Can you work these out from the drawing? Everything is in mm from the part's minimum corner. Round coordinates to 2 decimals unless told otherwise and drop trailing zeros. Write each loop counter-clockwise with the first axis right and the second up, starting at its lowest first coordinate (ties: lowest second). Pieces come first, ordered by that corner, then holes. Notation, with made-up numbers: M -28.5,13.25 L -24.5,13.25 A25 cw -24.5,43.25 Z; hole C 79,79.5 d1. An arc over 180 degrees is marked long. Use a Markdown table: item, result. Add a question column.
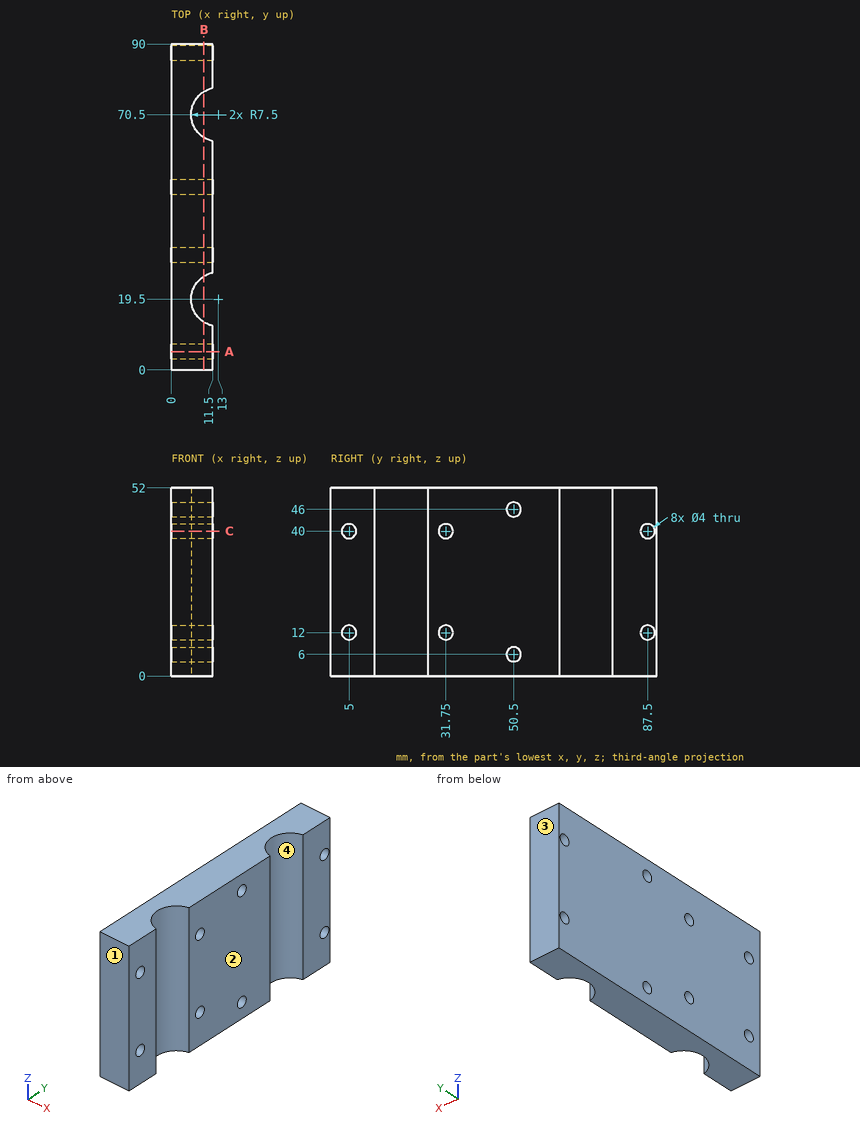
Item 1: Imagine slicing it at B-B on x = 9. Count the separate pieces of the cut face and the enclosed holes in it, plus the area to 3 significant figures.
Item 2: I need wall thicknesses on probe 1 along Z at (x, y) = (3.75, 50.5); probe 2 along Y at (x, z) = (11, 34); probe 3 along Y at (x, z) = (10.5, 34). Which ranges of each line are inside material? Lowest first, please. Write a range as from..to.
Item 3: Imagine slicing it at A-A on y = 5. List the corners of the cut face in (x, z) for me, plus the area to 3 significant figures.
Item 4: For pin 1 Ø1 at (y, z) = (69, 27) entering from +X, with a flat end and sliding along its axis, tell me the tip position at first contact or that it passes through.
Item 5: Imagine slicing it at C-C on z = 40. List the corners of the cut face in (x, y) for me.
Item 6: If we mould it in two halves opening along Y, with no side actions, what happens to the marked faces 1, 2, 3 and 4? For each: +Y half, -Y half, draft (parallel to the pull), parting line (faces both ways), or undercut.
The answers:
| question | item | result |
|---|---|---|
| 1 | separate pieces | 3 |
| 1 | enclosed holes | 8 |
| 1 | area | 3,260 mm² |
| 2 | probe 1 | 0..4, 8..44, 48..52 |
| 2 | probe 2 | 0..12.27, 26.73..63.27, 77.73..90 |
| 2 | probe 3 | 0..12.43, 26.57..63.43, 77.57..90 |
| 3 | outline | M 0,0 L 11.5,0 L 11.5,10 L 0,10 Z; M 0,14 L 11.5,14 L 11.5,38 L 0,38 Z; M 0,42 L 11.5,42 L 11.5,52 L 0,52 Z |
| 3 | area | 506 mm² |
| 4 | pin 1 | x = 5.77 |
| 5 | outline | M 0,0 L 11.5,0 L 11.5,3 L 0,3 Z; M 0,7 L 11.5,7 L 11.5,12.15 A7.5 cw 11.5,26.85 L 11.5,29.75 L 0,29.75 Z; M 0,33.75 L 11.5,33.75 L 11.5,63.15 A7.5 cw 11.5,77.85 L 11.5,85.5 L 0,85.5 Z; M 0,89.5 L 11.5,89.5 L 11.5,90 L 0,90 Z |
| 6 | face 1 | -Y half |
| 6 | face 2 | draft |
| 6 | face 3 | +Y half |
| 6 | face 4 | undercut |
